Solid Edge part; units mm, degrees
sketch "Sketch1" plane through (0, 0, 0) normal (1, 0, 0) x (0, 1, 0)
  line L0 (-59.6342, 10.695) -> (-59.6342, 48.795)
  line L1 (-59.6342, 48.795) -> (-59.6342, 61.495)
  line L2 (-59.6342, 61.495) -> (181.6658, 61.495)
  line L3 (181.6658, 61.495) -> (181.6658, 48.795)
  line L4 (181.6658, 10.695) -> (181.6658, 48.795)
  line L5 (175.3158, 10.695) -> (181.6658, 10.695)
  line L6 (168.6119, 17.3988) -> (175.3158, 10.695)
  line L7 (156.2658, 29.745) -> (168.6119, 17.3988)
  line L8 (137.2158, 10.695) -> (156.2658, 29.745)
  line L9 (-15.1842, 10.695) -> (137.2158, 10.695)
  line L10 (-15.1842, 10.695) -> (-34.2342, 29.745)
  line L11 (-34.2342, 29.745) -> (-53.2842, 10.695)
  line L12 (-53.2842, 10.695) -> (-59.6342, 10.695)
extrude "Protrusion1" add sketch "Sketch1" against normal blind 152.4
sketch "Sketch2" plane through (-76.2, -59.6342, 36.095) normal (0, -1, 0) x (1, 0, 0)
  line L0 (12.7, 25.4) -> (25.4, 12.7)
  line L1 (25.4, 12.7) -> (12.7, 12.7)
  line L2 (6.35, 12.7) -> (12.7, 12.7)
  line L3 (6.35, 6.35) -> (6.35, 12.7)
  line L4 (-6.35, 6.35) -> (6.35, 6.35)
  line L5 (-6.35, 12.7) -> (-6.35, 6.35)
  line L6 (-12.7, 12.7) -> (-6.35, 12.7)
  line L7 (-25.4, 12.7) -> (-12.7, 12.7)
  line L8 (-12.7, 25.4) -> (-25.4, 12.7)
  line L9 (-76.2, 25.4) -> (-12.7, 25.4)
extrude "Cutout1" cut sketch "Sketch2" against normal through all material side at (-57.1854, -59.6342, 55.1096)
sketch "Sketch3" plane through (-76.2, -59.6342, 36.095) normal (0, -1, 0) x (1, 0, 0)
  line L0 (76.2, -76.2) -> (-76.2, -76.2)
  line L1 (-76.2, -76.2) -> (-76.2, 25.4)
  line L2 (-76.2, 25.4) -> (76.2, 25.4)
  line L3 (76.2, 25.4) -> (76.2, -76.2)
extrude "ExtrudedProtrusion_2" add sketch "Sketch3" along normal blind 12.7
sketch "Sketch4" plane through (-76.2, 181.6658, 36.095) normal (0, 1, 0) x (-1, 0, 0)
  line L0 (-76.2, 25.4) -> (76.2, 25.4)
  line L1 (76.2, 25.4) -> (76.2, -25.4)
  line L2 (76.2, -25.4) -> (-76.2, -25.4)
  line L3 (-76.2, -25.4) -> (-76.2, 25.4)
extrude "ExtrudedProtrusion_3" add sketch "Sketch4" along normal blind 12.7
hole "Hole_1" at (-120.65, 61.0158, 61.495) direction (0, 0, -1) diameter 15.875 end up to next counterbore diameter 21.4325 counterbore depth 12.5984
hole "Hole1" at (-31.75, 61.0158, 61.495) direction (0, 0, -1) diameter 15.875 end up to next counterbore diameter 21.4325 counterbore depth 12.5984
Read the model definition and answer for the solid it produces. Units are mm, in the model's axes. A direction names the side the tool comes from. Coordinates: 2 decimals unless noted, no trailing zeros. Loops run counter-clockwise (first coordinate to the right, second up) from the corner with the lowest first, then second, coordinate; pieces in that order, holes last. Notation, with made-up numbers: (35, -32) -> (92, -32) arc R18 cw to (92, -16) -> close; hole circle Ø6 at (-19.5, 30.25). An arc over 180 degrees is marked (long way). Answer in a Markdown table with one row per item.
Item 1: A cutting plane is placed at B-B on y = 47.5. Determine the outline of the cut face in (x, z) (3 decimals), plus the area to 3 significant figures.
Returned:
| item | result |
|---|---|
| outline | (-152.4, 10.695) -> (0, 10.695) -> (0, 61.495) -> (-63.5, 61.495) -> (-50.8, 48.795) -> (-69.85, 48.795) -> (-69.85, 42.445) -> (-82.55, 42.445) -> (-82.55, 48.795) -> (-101.6, 48.795) -> (-88.9, 61.495) -> (-152.4, 61.495) -> close |
| area | 7,180 mm^2 |
Item 2: A cutting plane is placed at D-D on z = 53.5. Give the number of separate pieces and of enclosed holes in the cut face, plus the area to 3 significant figures.
Returned:
| item | result |
|---|---|
| separate pieces | 1 |
| enclosed holes | 3 |
| area | 29,900 mm^2 |
Item 3: For faces 1 (the flat face through (-82.55, 59, 46)), 2 (the flat face through (-75.13, -43.63, 20.35)), 3 (the flat face through (-75, -56, 10.695)), determine the directions among +Z, -Z, +X, -X, +Y, -Y from which every point of the face is accessible in a straight line to the end or side of a thin tool.
Returned:
| item | result |
|---|---|
| face 1 | +Z |
| face 2 | -Z, +X, -X |
| face 3 | -Z, +X, -X, +Y |
Item 4: A cutting plane is placed at C-C on x = -105.5. Determine the outline of the cut face in (y, z) (3 decimals), plus the area to 3 significant figures.
Returned:
| item | result |
|---|---|
| outline | (-72.334, -40.105) -> (-59.634, -40.105) -> (-59.634, 10.695) -> (-53.284, 10.695) -> (-34.234, 29.745) -> (-15.184, 10.695) -> (137.216, 10.695) -> (156.266, 29.745) -> (168.612, 17.399) -> (175.316, 10.695) -> (194.366, 10.695) -> (194.366, 61.495) -> (-72.334, 61.495) -> close |
| area | 13,500 mm^2 |
Item 5: Straight lines are drawn through the part: line 1 along Y through (x, z) = (-94.5, 54); line 2 along X through (y, z) = (135.5, 43.5); line 3 along Y through (x, z) = (-66, -14.5). For each, find the intervals that lie inside material, in ascending order. Write a range as [from, to].
Returned:
| item | result |
|---|---|
| line 1 | y = [-72.33, -59.63], [181.67, 194.37] |
| line 2 | x = [-152.4, -82.55], [-69.85, 0] |
| line 3 | y = [-72.33, -59.63] |
Item 6: Each of these flat-tipped pins is pushed along its axis until it touches: P1, Ø7, axis at x = -59.5, y = -57, coming from the -Z side (3 decimals); P2, Ø10.5, axis at x = -121, y = 61, coming from the +Z side; P3, Ø5, axis at x = -38, y = -13.5, coming from the -Z side (3 decimals); P4, Ø14, axis at x = -75, y = 98.5, coming from the +Z side (3 decimals). Where does it stop, or does it pass through?
Returned:
| item | result |
|---|---|
| P1 | stops at z = -40.105 |
| P2 | passes through |
| P3 | stops at z = 10.695 |
| P4 | stops at z = 48.795 |
Item 7: A cutting plane is placed at A-A on x = -31.75. Determine the outline of the cut face in (y, z) (3 decimals), plus the area to 3 significant figures.
Returned:
| item | result |
|---|---|
| outline | (-72.334, -40.105) -> (-59.634, -40.105) -> (-59.634, 10.695) -> (-53.284, 10.695) -> (-34.234, 29.745) -> (-15.184, 10.695) -> (53.078, 10.695) -> (53.078, 48.897) -> (50.3, 48.897) -> (50.3, 61.495) -> (-72.334, 61.495) -> close; (68.953, 10.695) -> (137.216, 10.695) -> (156.266, 29.745) -> (168.612, 17.399) -> (175.316, 10.695) -> (194.366, 10.695) -> (194.366, 61.495) -> (71.732, 61.495) -> (71.732, 48.897) -> (68.953, 48.897) -> close |
| area | 12,600 mm^2 |
Item 8: For a pull along Z with two mould halves and no side action, classify faces 4 (the flat face through (-76, 59, 42.445)), 5 (the flat face through (-92, 59, 48.795)), 6 (the cylindrical face through (-113.957, 56.749, 30.063)), 7 (the flat face through (-75.13, 146.61, 20.09)) as released by +Z, released by -Z, zero draft, split by the parting line, or undercut.
Returned:
| item | result |
|---|---|
| face 4 | released by +Z |
| face 5 | undercut |
| face 6 | zero draft |
| face 7 | released by -Z |
